from build123d import *

# Parameters (mm, degrees)
SKETCH2_R           = 15
BOSS_EXTRUDE1_DEPTH = 20


with BuildPart() as part:
    # Sketch2 → Boss-Extrude1 (new, symmetric)
    with BuildSketch(Plane.XY):
        with BuildLine():
            Line((0, 0), (-150, 0))
            Line((-150, 0), (-150, 20))
            Line((-150, 20), (-115, 20))
            Line((-115, 20), (-115, 15))
            Line((-115, 15), (-90, 15))
            Line((-90, 15), (-90, 20))
            Line((-90, 20), (-60, 20))
            Line((-60, 20), (-60, 40))
            ThreePointArc((-60, 40), (-30, 70), (0, 40))
            Line((0, 40), (0, 0))
        make_face()
        with Locations((-30, 40)):
            Circle(SKETCH2_R, mode=Mode.SUBTRACT)
    extrude(amount=BOSS_EXTRUDE1_DEPTH, both=True)


solid = part.part
CAD build for the part. Positions are in the model's coordinates, mm. A direction names the side the tool comes from. Round coordinates to 2 decimals unless told otherwise and drop trailing zeros. Order: outer loops, then holes, each group sorted by start corner. A loop starts at its lowest first (then second) coordinate and runs counter-clockwise, first axis right, second up. Notation, with made-up numbers: (68, 12) -> (109, 12) arc R18 cw to (109, 23) -> close; hole circle Ø6 at (-10.5, 37.5). An arc over 180 degrees is marked (long way). Write item = value, one per line. Start each with the question number.
(1) Which spindle directions (+Z, -Z, +X, -X, +Y, -Y) get a long thin tool onto all of the face, cutting with end or side? Do faces 1 (the flat face through (-60, 30, 0)), 2 (the flat face through (-90, 17, 0)), 3 (the flat face through (0, 20, 0)). Say none if no direction does.
(2) Cut at B-B, the plane z = 0. List the corners of the cut face in (x, y), then the cut area to 3 significant figures.
(3) Cut at C-C, the plane y = 48. List the corners of the cut face in (x, z), then the cut area to 3 significant figures.
(4) Probe line 1 (Y direction, x = -30, z = -9); line 2 (Y direction, x = -114.5, z = 4); line 3 (Y direction, x = -121.5, z = -8.5). List the from-to ranges inside material, lowest first. Write a range as [from, to].
(5) Cut at D-D, the plane x = -131.5. List the corners of the cut face in (y, z), then the cut area to 3 significant figures.
(6) Cut at A-A, the plane x = -30. List the corners of the cut face in (y, z).
(7) Pin check, flat tips, straight feed: P1, Ø1.5, axis at y = 42.5, z = 15.5, coming from the -X side; P2, Ø1, axis at x = -15.5, z = -3.5, coming from the +Y side; P3, Ø18, axis at x = -30, y = 40, coming from the +Z side; P4, Ø12.5, axis at x = -96.5, z = -7.5, coming from the +Y side. Stop position of each tip, or through.
(8) Pull direction X, two halves, no side cores. Call faces 4 (the cylindrical face through (-30.66, 69.993, 0.28)), 5 (the flat face through (-115, 18, 0)), 6 (the flat face through (-75, 20, 0)): released by +X, released by -X, zero draft, split by the parting line, or undercut.
Model answer:
q1.face_1 = +Z, -Z, -X, +Y
q1.face_2 = +Z, -Z, +Y
q1.face_3 = +Z, -Z, +X, +Y, -Y
q2.outline = (-150, 0) -> (0, 0) -> (0, 40) arc R30 ccw to (-60, 40) -> (-60, 20) -> (-90, 20) -> (-90, 15) -> (-115, 15) -> (-115, 20) -> (-150, 20) -> close; hole circle Ø30 at (-30, 40)
q2.area = 4,780 mm2
q3.outline = (-58.91, -20) -> (-42.69, -20) -> (-42.69, 20) -> (-58.91, 20) -> close; (-17.31, -20) -> (-1.09, -20) -> (-1.09, 20) -> (-17.31, 20) -> close
q3.area = 1,300 mm2
q4.line_1 = [0, 25], [55, 70]
q4.line_2 = [0, 15]
q4.line_3 = [0, 20]
q5.outline = (0, -20) -> (20, -20) -> (20, 20) -> (0, 20) -> close
q5.area = 800 mm2
q6.outline = (0, -20) -> (25, -20) -> (25, 20) -> (0, 20) -> close; (55, -20) -> (70, -20) -> (70, 20) -> (55, 20) -> close
q7.P1 = -59.95
q7.P2 = 66.53
q7.P3 = through
q7.P4 = 15
q8.face_4 = split by the parting line
q8.face_5 = undercut
q8.face_6 = zero draft
